Input: part model. Units: mm. Frame: model coordinates. Give positions to 0.01 mm unless a question says otherwise; leave off trailing zeros. Loops run counter-clockwise (first coordinate to the right, second up) from the corner with the lowest first, then second, coordinate; pieces in that order, holes last. Notation, with made-up numbers: (86, 17) - (102, 17) arc R23 cw to (102, 26) - close; hole circle Ø4 at (-0.75, 7). An arc over 180 degrees is marked (long way). Answer as a JSON object with one key per item and string values. Group by question number.
(1) Pin query (flat end, axial travel): P1, Ø1, axis at x = 11.5, z = 69, coming from the -Y side; P2, Ø5, axis at y = -1, z = 26, coming from the -X side; P3, Ø5, axis at y = -20, z = 25.5, coming from the -X side. Return the tip coordinate at first contact, or that it passes through.
(2) Section query B-B (x = -10.5). Return loops of the section in (y, z).
(3) Section query C-C (y = 3). Return loops of the section in (x, z).
(4) Section query D-D (z = 88). Return loops of the section in (x, y), plus the area to 3 significant figures.
(5) Section query A-A (z = 105). Return loops of the section in (x, y).
(6) Material intervals for L1, parallel to Y at x = -13, z = 19; L2, parallel to Y at x = -5.5, z = 26; L3, parallel to X at y = 8.5, z = 30, sorted ascending.
```python
from build123d import *


with BuildPart() as f3:
    # F0 (on Top) → F3 section 0
    with BuildSketch(Plane.XY, mode=Mode.PRIVATE) as f3_s0:
        Polygon((-32.177303, 8.740868), (-32.177303, 0), (0, -35.571251), (30.187905, 0), (30.187905, 8.740868), (20.614294, 16.399754), (-22.056634, 16.399754), align=None)
    loft([f3_s0.sketch, Vertex(0, 5.783991, 127)])


solid = f3.part
```
Recorded:
{
 "1": {"P1": "stops at y = -0.16", "P2": "stops at x = -25.92", "P3": "stops at x = -8.95"},
 "2": {"outline": "(-23.96, 0) - (16.4, 0) - (10.84, 66.54) - (6.75, 85.56) - (3.9, 85.56) - close"},
 "3": {"outline": "(-32.18, 0) - (30.19, 0) - (14.53, 65.87) - (0, 118.45) - (-15.49, 65.87) - close"},
 "4": {"outline": "(-9.88, 4.01) - (0, -6.92) - (9.27, 4.01) - (9.27, 6.69) - (6.33, 9.04) - (-6.77, 9.04) - (-9.88, 6.69) - close", "area": "194 mm^2"},
 "5": {"outline": "(-5.57, 4.78) - (0, -1.38) - (5.23, 4.78) - (5.23, 6.3) - (3.57, 7.62) - (-3.82, 7.62) - (-5.57, 6.3) - close"},
 "6": {"L1": "y = -15.01 to 14.81", "L2": "y = -21.02 to 14.23", "L3": "x = -23.97 to 22.48"}
}
